Check sheet for the modelled part. Datum: model origin and axes. Units: mm. Face numbers are marked on the shaded views. Give positions to 0.01 mm unless a question says otherwise; leave off trailing zeros. Order: outer loops, then holes, each group sorted by start corner. A loop starts at its lowest first (then second) coordinate and runs counter-clockwise, first axis right, second up. Notation, with made-up numbers: M -38,-19.75 L -26,-19.75 A12 cw -26,-4.75 Z; hole C 9,33.25 d11. An arc over 180 degrees is marked long. Return JSON: item names as keys, results as strings. Group by question number.
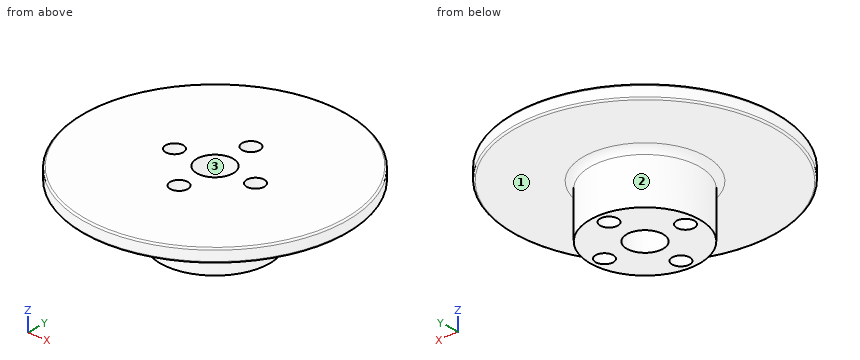
Autodesk Inventor part; units mm, degrees
ref_plane "YZ Plane" through (0, 0, 0) normal (1, 0, 0) x (0, 1, 0)
ref_plane "XZ Plane" through (0, 0, 0) normal (0, 1, 0) x (-1, 0, 0)
ref_plane "XY Plane" through (0, 0, 0) normal (0, 0, 1) x (1, 0, 0)
sketch "Sketch1" plane through (0, 0, 0) normal (0, 1, 0) x (-1, 0, 0)
  line L0 (0, 0) -> (25.0825, 0)
  line L1 (25.0825, -25.4) -> (0, -25.4)
  line L2 (0, -25.4) -> (0, 0)
  line L3 (25.0825, -2.54) -> (11.8039, -2.54)
  line L4 (25.0825, -22.86) -> (11.8039, -22.86)
  line L5 (10.5339, -3.81) -> (10.5339, -21.59)
  line L6 (25.4, -0.3175) -> (25.4, -2.2225)
  line L7 (25.4, -23.1775) -> (25.4, -25.0825)
  arc A0 (25.4, -0.3175) -> (25.0825, 0) centre (25.0825, -0.3175) ccw
  arc A1 (25.0825, -2.54) -> (25.4, -2.2225) centre (25.0825, -2.2225) ccw
  arc A2 (25.4, -23.1775) -> (25.0825, -22.86) centre (25.0825, -23.1775) ccw
  arc A3 (25.0825, -25.4) -> (25.4, -25.0825) centre (25.0825, -25.0825) ccw
  arc A4 (11.8039, -2.54) -> (10.5339, -3.81) centre (11.8039, -3.81) ccw
  arc A5 (10.5339, -21.59) -> (11.8039, -22.86) centre (11.8039, -21.59) ccw
  point P0 (25.4, -25.4)
  point P1 (25.4, 0)
  dimension "d0" = 25.4
  dimension "d2" = 2.54
  dimension "d3" = 2.54
  dimension "d4" = 0.3175
  dimension "d5" = 1.27
  dimension "d7" = 25.4
revolve "Revolution1" add sketch "Sketch1" angle 360 about axis through (0, 0, -25.4) along (0, 0, 1)
sketch "Sketch2" plane through (0, 0, 0) normal (0, 0, 1) x (1, 0, 0)
  circle A0 centre (0, 0) radius 3.5
  circle A1 centre (0, 8) radius 1.7
  circle A2 centre (0, 0) radius 8
  circle A3 centre (-8, 0) radius 1.7
  circle A4 centre (0, -8) radius 1.7
  circle A5 centre (8, 0) radius 1.7
  dimension "d10" = 16
  dimension "d8" = 7
  dimension "d9" = 3.4
  dimension "d13" = 360
extrude "Extrusion1" cut sketch "Sketch2" against normal through all contours A0 | A1 A2 | A2 A1 | A3 A2 | A2 A3 | A5 A2 | A2 A5 | A4 A2 | A2 A4
ref_plane "Work Plane1" through (0, 0, -12.7) normal (0, 0, -1) x (-1, 0, 0)
sketch "Sketch3" plane through (0, 0, -25.4) normal (0, 0, -1) x (-1, 0, 0)
  circle A0 centre (0, 0) radius 25.4
  point P0 (0, 0)
extrude "Extrusion2" cut sketch "Sketch3" against normal blind 12.7
properties part number "Pulley"
1) Depth check by flat-ended pin: P1, Ø25, axis at x = -10.5, y = 4.5, coming from the -Z side; P2, Ø5, axis at x = 3.5, z = -3.5, coming from the +Y side; P3, Ø3, axis at x = -7, z = -2.5, coming from the +Y side; P4, Ø3, axis at x = 0, y = 8, coming from the -Z side. Enter the tip coordinate at first touch or a pass-through.
2) Material ranges on line 1 along Y through (x, z) = (0, -9.75); line 2 along Z through (x, y) = (15, -12.5); line 3 along X through (y, z) = (2, -3.75), recorded low to high.
3) Sectioned sample at B-B on z = -5. Record the boundary of the cut face in (x, y).
4) Sectioned sample at A-A on x = 0. Record the boundary of the cut face in (y, z) (1 decimal), then the cut area to 3 significant figures.
5) Release check for a two-part mould opening along X. For the marked faces 1, 2 and 3 record: released by +X, released by -X, zero draft, split by the parting line, or undercut.
Reply:
{
 "1": {"P1": "z = -12.7", "P2": "y = 25.36", "P3": "y = 24.79", "P4": "through"},
 "2": {"line 1": "-10.53 to -9.7, -6.3 to -3.5, 3.5 to 6.3, 9.7 to 10.53", "line 2": "-2.54 to 0", "line 3": "-10.34 to -2.87, 2.87 to 10.34"},
 "3": {"outline": "C 0,0 d21.07; hole C -8,0 d3.4; hole C 0,0 d7; hole C 0,-8 d3.4; hole C 0,8 d3.4; hole C 8,0 d3.4"},
 "4": {"outline": "M -25.4,-2.2 A0.3 ccw -25.1,-2.5 L -11.8,-2.5 A1.3 cw -10.5,-3.8 L -10.5,-12.7 L -9.7,-12.7 L -9.7,0 L -25.1,0 A0.3 ccw -25.4,-0.3 Z; M -6.3,-12.7 L -3.5,-12.7 L -3.5,0 L -6.3,0 Z; M 3.5,-12.7 L 6.3,-12.7 L 6.3,0 L 3.5,0 Z; M 9.7,-12.7 L 10.5,-12.7 L 10.5,-3.8 A1.3 cw 11.8,-2.5 L 25.1,-2.5 A0.3 ccw 25.4,-2.2 L 25.4,-0.3 A0.3 ccw 25.1,0 L 9.7,0 Z", "area": "168 mm^2"},
 "5": {"face 1": "zero draft", "face 2": "split by the parting line", "face 3": "undercut"}
}
